Design review of the part built by this model. Coordinates are the model's own, in mm. Face numbers are marked on the shaded views. Coordinates: 2 decimals unless noted, no trailing zeros. Write each loop counter-clockwise with the first axis right and the second up, starting at its lowest first coordinate (ties: lowest second). Pieces come first, ordered by that corner, then holes. Notation, with made-up numbers: (62.5, 16.5) -> (86.5, 16.5) arc R22 ccw to (86.5, 49.5) -> close; hole circle Ø7 at (32, 30). An arc over 180 degrees is marked (long way). Answer in a Markdown table with one row per item. Add a question column.
Item 1: Take a section at A-A, the plane z = 4.75. Write out the cut boundary in (x, y).
Item 2: Clearance check with flat-ended pins moving along their axes: P1, Ø1, axis at y = -1, z = 6, coming from the +X side; P2, Ø5, axis at y = -2.5, z = 7, coming from the +X side; P3, Ø3, axis at x = -1, z = 10, coming from the -Y side. State where each tip first meets the part, or that it passes through.
Item 3: Take a section at B-B, the plane x = 2.25. Give the number of separate pieces and of enclosed holes in the cut face, and give its area (3 significant figures).
Item 4: To check wall thickness, follow line 1 (Z direction, x = 2.75, y = 1.25); line 2 (X direction, y = -0.75, z = 1); line 3 (X direction, y = 1.5, z = 12.5). State the ranges of each line that lie inside material, in increasing order.
Item 5: Draft analysis for pull direction X (two halves, no side actions). For the marked faces 1, 2, 3 and 4, state which applies: released by +X, released by -X, zero draft, split by the parting line, or undercut.
from build123d import *

# Parameters (mm, degrees)
SCHIZZO1_R                   = 4.25
ESTRUSIONE_ESTRUSIONE1_DEPTH = 5
SCHIZZO2_R                   = 2.5
ESTRUSIONE_ESTRUSIONE2_DEPTH = 14
TAGLIO_ESTRUSIONE1_DEPTH     = 2.5
RACCORDO1_R                  = 0.25
RACCORDO2_R                  = 0.2
SMUSSO1_SIZE                 = 0.445
RIPETIZIONE_A_L1_COUNT       = 13
RIPETIZIONE_A_L1_PITCH       = 0.844


with BuildPart() as part:
    # Schizzo1 → Estrusione-Estrusione1 (new body)
    with BuildSketch(Plane.XY):
        Circle(SCHIZZO1_R)
    extrude(amount=ESTRUSIONE_ESTRUSIONE1_DEPTH)

    # Schizzo2 → Estrusione-Estrusione2 (add)
    with BuildSketch(Plane.XY.offset(5)):
        Circle(SCHIZZO2_R)
    extrude(amount=ESTRUSIONE_ESTRUSIONE2_DEPTH)

    # Schizzo3 → Taglio-Estrusione1 (cut)
    with BuildSketch(Plane(origin=(0, 0, 0), x_dir=(-1, 0, 0), z_dir=(0, 0, -1))):
        Polygon((0, 2.358), (-2.042087902, 1.179), (-2.042087902, -1.179), (0, -2.358), (2.042087902, -1.179), (2.042087902, 1.179), align=None)
    extrude(amount=-TAGLIO_ESTRUSIONE1_DEPTH, mode=Mode.SUBTRACT)

    # Raccordo1
    raccordo1_edges = [part.edges().sort_by_distance(p)[0] for p in [
        (-4.25, 0, 0),
    ]]
    fillet(raccordo1_edges, radius=RACCORDO1_R)

    # Raccordo2
    raccordo2_edges = [part.edges().sort_by_distance(p)[0] for p in [
        (-2.5, 0, 5),
    ]]
    fillet(raccordo2_edges, radius=RACCORDO2_R)

    # Smusso1
    smusso1_edges = [part.edges().sort_by_distance(p)[0] for p in [
        (-2.5, 0, 19),
    ]]
    chamfer(smusso1_edges, length=SMUSSO1_SIZE)

    # Schizzo4 → Taglia-Rivoluzione1 (revolve, cut)
    with BuildSketch(Plane(origin=(0, 0, 0), x_dir=(0, 0, -1), z_dir=(1, 0, 0))):
        Polygon((-7.945118296, -2.055), (-8.25671065, -2.5), (-8.25671065, -3.125), (-7.633525941, -3.125), (-7.633525941, -2.5), align=None)
    taglia_rivoluzione1 = revolve(axis=Axis((0, 0, 0), (0, 0, 1)), mode=Mode.SUBTRACT)

    # Ripetizione a L1: Taglia-Rivoluzione1 ×13
    with Locations(*[(0, 0, i * RIPETIZIONE_A_L1_PITCH) for i in range(1, RIPETIZIONE_A_L1_COUNT)]):
        add(taglia_rivoluzione1, mode=Mode.SUBTRACT)

    # Schizzo5 → Taglia-Rivoluzione2 (revolve, cut)
    with BuildSketch(Plane(origin=(0, 0, 0), x_dir=(0, 0, -1), z_dir=(1, 0, 0))):
        Polygon((0, -2.042), (-2.5, -2.042), (-3.67894925, 0), (0, 0), align=None)
    revolve(axis=Axis((0, 0, 3.67894925), (0, 0, -1)), mode=Mode.SUBTRACT)


solid = part.part
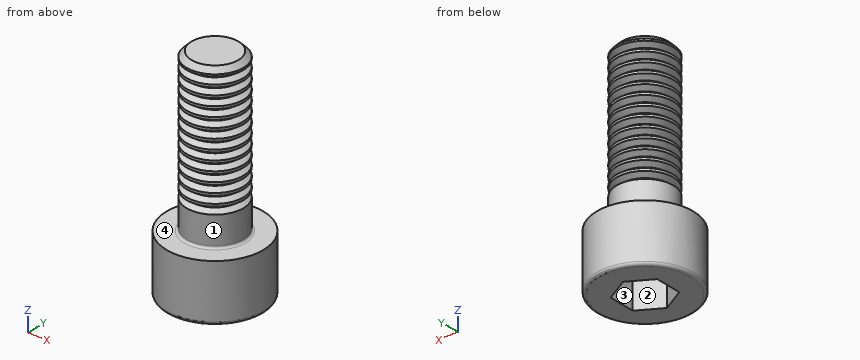
Answers:
| question | item | result |
|---|---|---|
| 1 | outline | circle Ø8.5 at (0, 0) |
| 2 | P1 | stops at x = 2.45 |
| 2 | P2 | stops at x = 4.13 |
| 2 | P3 | stops at y = -2.5 |
| 3 | separate pieces | 14 |
| 3 | enclosed holes | 0 |
| 3 | area | 54.8 mm^2 |
| 4 | line 1 | z = 0 to 5 |
| 4 | line 2 | x = -4.18 to -2.04, 2.04 to 4.18 |
| 4 | line 3 | x = -2 to 2 |
| 5 | face 1 | split by the parting line |
| 5 | face 2 | undercut |
| 5 | face 3 | undercut |
| 5 | face 4 | zero draft |
